The figure shows three views and two pictorial views of one solid part (mm, origin at its lowest corner). Answer the questions. Round coordinates to 2 decimals unless told otherwise and drop trailing zeros. Write each loop counter-clockwise with the first axis right and the second up, starting at its lowest first coordinate (ties: lowest second). Pieces come first, ordered by that corner, then holes. Notation, with made-up numbers: M -36,13 L -8,13 A25 cw -8,36 Z; hole C -19.5,66 d5. An arc over 180 degrees is marked long. One line per item, written item: value. Start each with the question number.
Q1. Find section B-B (y = 2.05). Write down the section's boundary in (x, z).
Q2. Find section A-A (z = 92.5). Write down the section's boundary in (x, y), and give its area (3 significant figures).
Q3. Find section C-C (x = 84.5). Write down the section's boundary in (y, z), and give its area (3 significant figures).
Q4. Consider probe 1 along Z at (x, y) = (51, 0.7); probe 2 along X at (y, z) = (1.55, 38.5). Determine where each line is inside the solid, lowest interval first.
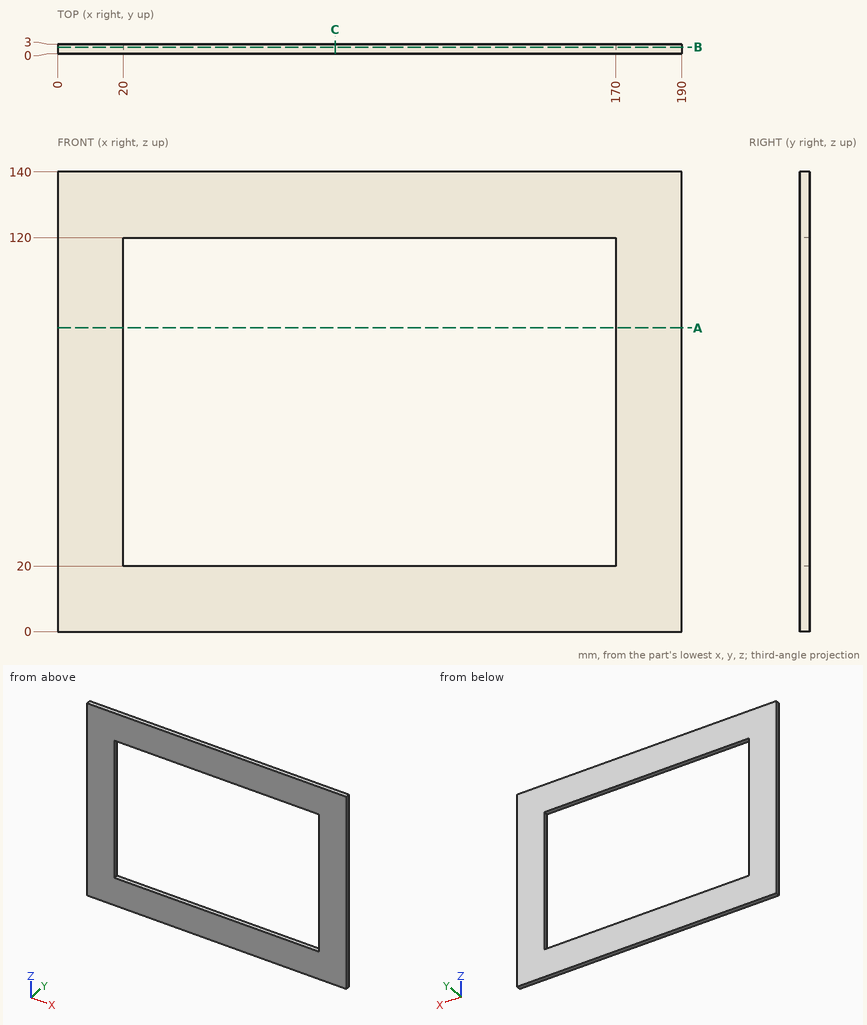
The answers:
1. outline: M 0,0 L 190,0 L 190,140 L 0,140 Z; hole M 20,20 L 170,20 L 170,120 L 20,120 Z
2. outline: M 0,0 L 20,0 L 20,3 L 0,3 Z; M 170,0 L 190,0 L 190,3 L 170,3 Z
2. area: 120 mm2
3. outline: M 0,0 L 3,0 L 3,20 L 0,20 Z; M 0,120 L 3,120 L 3,140 L 0,140 Z
3. area: 120 mm2
4. probe 1: 0 to 20, 120 to 140
4. probe 2: 0 to 20, 170 to 190
